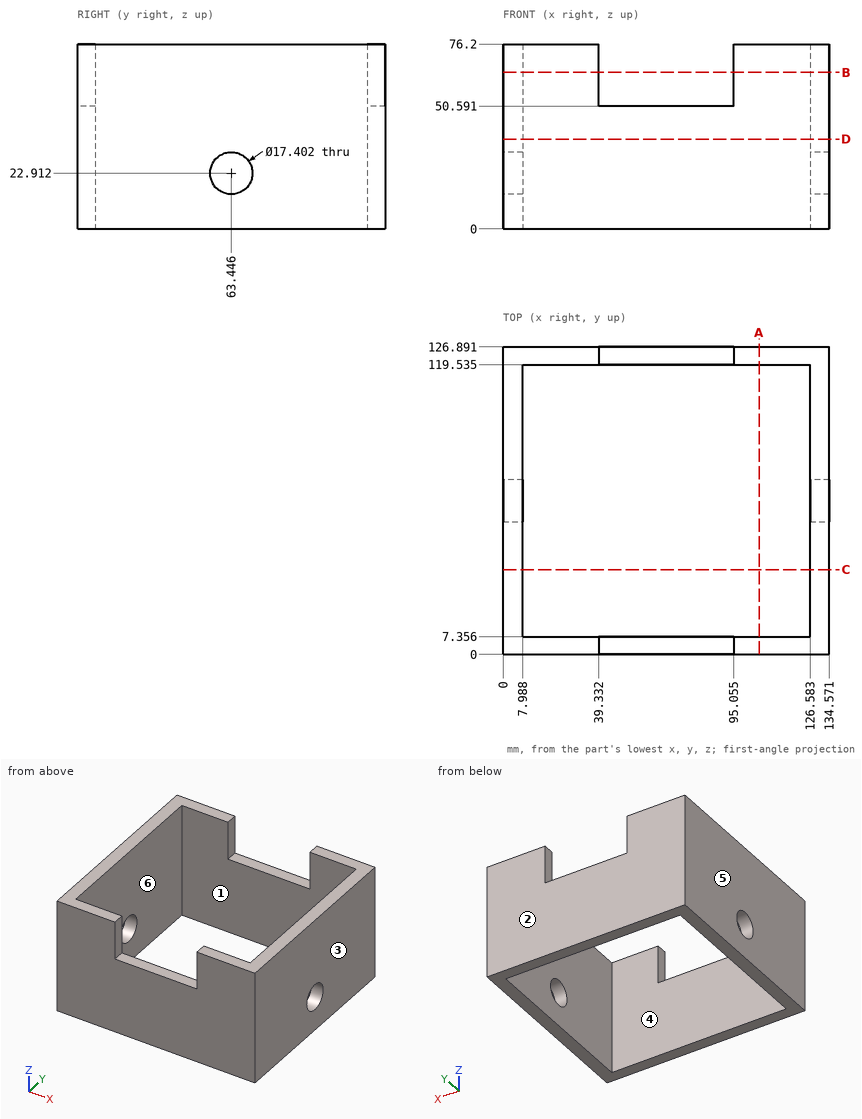
Job drawing, mm, ordinate dimensions from the low corner. One solid piece. A direction names the side the tool comes from. Give positions to 0.01 mm unless a question says otherwise; leave off trailing zeros. Loops run counter-clockwise (first coordinate to the right, second up) from the corner with the lowest first, then second, coordinate; pieces in that order, holes last. Notation, with made-up numbers: M 11,0.5 L 41,0.5 A19 ccw 41,26.5 Z; hole C 54.25,43 d8. An arc over 180 degrees is marked long. Return JSON: item names as keys, results as strings.
1) 3-axis set-ups, long thin cutter, end or side, ignore diameter. For the marked faces 5 and 6: which of +Z, -Z, +X, -X, +Y, -Y reach the whole face in a straight line?
Calculated:
{"face 5": "+Z, -Z, -X, +Y, -Y", "face 6": "+Z, -Z"}
2) Saw through at D-D, the plane z = 37. List the corners of the cut face in (x, y) (1 decimal), then the cut area to 3 significant figures.
Calculated:
{"outline": "M 0,0 L 134.6,0 L 134.6,126.9 L 0,126.9 Z; hole M 8,7.4 L 126.6,7.4 L 126.6,119.5 L 8,119.5 Z", "area": "3,770 mm2"}
3) Saw through at B-B, the plane z = 64.5. List the corners of the cut face in (x, y) (1 decimal).
Calculated:
{"outline": "M 0,0 L 39.3,0 L 39.3,7.4 L 8,7.4 L 8,119.5 L 39.3,119.5 L 39.3,126.9 L 0,126.9 Z; M 95.1,0 L 134.6,0 L 134.6,126.9 L 95.1,126.9 L 95.1,119.5 L 126.6,119.5 L 126.6,7.4 L 95.1,7.4 Z"}
4) Drill centre lines: line 1 (X direction, y = 24.5, z = 54); line 2 (Y direction, x = 57.5, z = 21) (1 decimal). Where is each one in solid material? Low to high.
Calculated:
{"line 1": "x = 0 to 7.99, 126.58 to 134.57", "line 2": "y = 0 to 7.4, 119.5 to 126.9"}
5) Saw through at C-C, the plane y = 35. List the corners of the cut face in (x, z).
Calculated:
{"outline": "M 0,0 L 7.99,0 L 7.99,76.2 L 0,76.2 Z; M 126.58,0 L 134.57,0 L 134.57,76.2 L 126.58,76.2 Z"}
6) Pull direction X, two halves, no side cores. Call the marked faces 1, 2, 3 and 4: released by +X, released by -X, zero draft, split by the parting line, or undercut.
Calculated:
{"face 1": "undercut", "face 2": "zero draft", "face 3": "released by +X", "face 4": "undercut"}
7) Saw through at A-A, the plane x = 105.5. List the corners of the cut face in (y, z) (1 decimal).
Calculated:
{"outline": "M 0,0 L 7.4,0 L 7.4,76.2 L 0,76.2 Z; M 119.5,0 L 126.9,0 L 126.9,76.2 L 119.5,76.2 Z"}
8) Flat gauge pins, fed straight in: pin 1 Ø5 at (x, z) = (40, 62) entering from -Y; pin 2 Ø6 at (x, y) = (57.5, 122) entering from +Z. Where does each tip first touch, or does it go through?
Calculated:
{"pin 1": "stops at y = 0", "pin 2": "stops at z = 50.59"}
